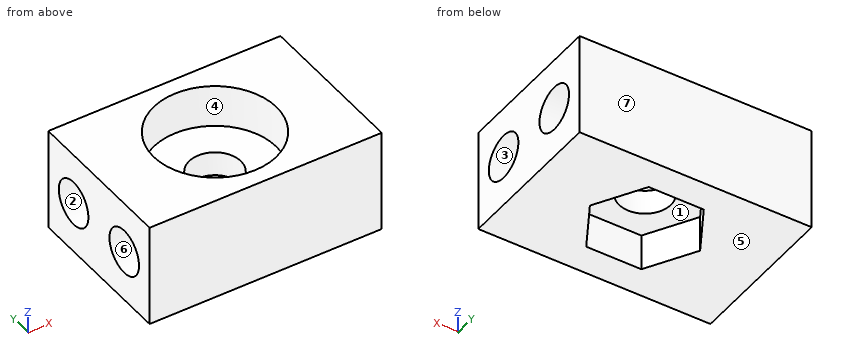
Autodesk Fusion 360 part; units mm, degrees
sketch "Sketch1" plane through (0, 0, 0) normal (0, 0, 1) x (1, 0, 0)
  line L0 (-9, -6) -> (9, -6)
  line L1 (9, -6) -> (9, 6)
  line L2 (9, 6) -> (-9, 6)
  line L3 (-9, 6) -> (-9, -6)
  dimension "d1" = 18
  dimension "d2" = 12
  dimension "d5" = 9
  dimension "d6" = 6
extrude "Extrude1" add sketch "Sketch1" along normal blind 8
sketch "Sketch2" plane through (0, 0, 0) normal (0, 0, -1) x (1, 0, 0)
  line L0 (-9, 6) -> (-9, -6)
  line L1 (-9, -6) -> (9, -6)
  line L2 (9, -6) -> (9, 6)
  line L3 (9, 6) -> (-9, 6)
sketch "Sketch3" plane through (0, 0, 0) normal (0, 0, -1) x (1, 0, 0)
  line L0 (2.1362, -3.7) -> (4.2724, 0)
  line L1 (4.2724, 0) -> (2.1362, 3.7)
  line L2 (2.1362, 3.7) -> (-2.1362, 3.7)
  line L3 (-2.1362, 3.7) -> (-4.2724, 0)
  line L4 (-4.2724, 0) -> (-2.1362, -3.7)
  line L5 (-2.1362, -3.7) -> (2.1362, -3.7)
  dimension "d12" = 3.7
extrude "Extrude2" cut sketch "Sketch3" against normal blind 2.8
sketch "Sketch4" plane through (0, 0, 8) normal (0, 0, 1) x (-1, 0, 0)
  line L0 (9, -6) -> (9, 6)
  line L1 (9, 6) -> (-9, 6)
  line L2 (-9, 6) -> (-9, -6)
  line L3 (-9, -6) -> (9, -6)
  circle A0 centre (0, 0) radius 2
  dimension "d9" = 4
extrude "Extrude3" cut sketch "Sketch4" against normal blind 10 contours A0
sketch "Sketch5" plane through (0, 0, 8) normal (0, 0, 1) x (-1, 0, 0)
  circle A0 centre (0, 0) radius 2
  line L0 (9, -6) -> (9, 6)
  line L1 (9, 6) -> (-9, 6)
  line L2 (-9, 6) -> (-9, -6)
  line L3 (-9, -6) -> (9, -6)
  circle A1 centre (0, 0) radius 4.75
  dimension "d21" = 9.5
extrude "Extrude4" cut sketch "Sketch5" against normal blind 3.3 contours A1
sketch "Sketch6" plane through (9, 0, 0) normal (1, 0, 0) x (0, 1, 0)
  line L0 (-6, 0) -> (6, 0)
  line L1 (6, 0) -> (6, 8)
  line L2 (6, 8) -> (-6, 8)
  line L3 (-6, 8) -> (-6, 0)
  line L4 (-6, 4) -> (6, 4) construction
  circle A0 centre (-3, 4) radius 1.75
  circle A1 centre (3, 4) radius 1.75
  dimension "d15" = 3.5
  dimension "d16" = 3.5
  dimension "d17" = 3
  dimension "d18" = 3
extrude "Extrude5" cut sketch "Sketch6" against normal blind 4.2 contours A0 | A1
sketch "Sketch7" plane through (-9, 0, 0) normal (-1, 0, 0) x (0, -1, 0)
  line L0 (-6, 0) -> (6, 0)
  line L1 (6, 0) -> (6, 8)
  line L2 (6, 8) -> (-6, 8)
  line L3 (-6, 8) -> (-6, 0)
  line L4 (-6, 4) -> (6, 4) construction
  circle A0 centre (-3, 4) radius 1.75
  circle A1 centre (3, 4) radius 1.75
  dimension "d24" = 3.5
  dimension "d25" = 3.5
  dimension "d26" = 3
  dimension "d27" = 3
extrude "Extrude6" cut sketch "Sketch7" against normal blind 4.2 contours A0 | A1
Could you check a few things on this model? Use its own coordinates, in mm. Face numbers are marked on the shaded views. A direction names the side the tool comes from. Give positions to 0.01 mm unless a question says otherwise; leave off trailing zeros. Loops run counter-clockwise (first coordinate to the right, second up) from the corner with the lowest first, then second, coordinate; pieces in that order, holes last. Notation, with made-up numbers: (39, 85.25) -> (91, 85.25) arc R12 ccw to (91, 97.25) -> close; hole circle Ø3 at (84.5, 56). An arc over 180 degrees is marked (long way). Return JSON: item names as keys, results as strings.
Item 1: If we section it at A-A on z = 4: List the corners of the cut face in (x, y) for me, plus the area to 3 significant figures.
Geometry results:
{"outline": "(-9, -6) -> (9, -6) -> (9, -4.75) -> (4.8, -4.75) -> (4.8, -1.25) -> (9, -1.25) -> (9, 1.25) -> (4.8, 1.25) -> (4.8, 4.75) -> (9, 4.75) -> (9, 6) -> (-9, 6) -> (-9, 4.75) -> (-4.8, 4.75) -> (-4.8, 1.25) -> (-9, 1.25) -> (-9, -1.25) -> (-4.8, -1.25) -> (-4.8, -4.75) -> (-9, -4.75) -> close; hole circle Ø4 at (0, 0)", "area": "145 mm²"}
Item 2: If we section it at D-D on x = -5.25: List the corners of the cut face in (y, z) for me.
Geometry results:
{"outline": "(-6, 0) -> (6, 0) -> (6, 8) -> (-6, 8) -> close; hole circle Ø3.5 at (-3, 4); hole circle Ø3.5 at (3, 4)"}
Item 3: If we section it at C-C on y = 0.25: List the corners of the cut face in (x, z) for me.
Geometry results:
{"outline": "(-9, 0) -> (-4.13, 0) -> (-4.13, 2.8) -> (-1.98, 2.8) -> (-1.98, 4.7) -> (-4.74, 4.7) -> (-4.74, 8) -> (-9, 8) -> close; (1.98, 2.8) -> (4.13, 2.8) -> (4.13, 0) -> (9, 0) -> (9, 8) -> (4.74, 8) -> (4.74, 4.7) -> (1.98, 4.7) -> close"}
Item 4: Which directions (+Z, -Z, +X, -X, +Y, -Y) give clear straight access to the entire face, cutting with the end or side of a thin tool? Please do the marked faces 1, 2, 3 and 4.
Geometry results:
{"face 1": "-Z", "face 2": "-X", "face 3": "+X", "face 4": "+Z"}
Item 5: If we section it at B-B on x = 0: List the corners of the cut face in (y, z) for me.
Geometry results:
{"outline": "(-6, 0) -> (-3.7, 0) -> (-3.7, 2.8) -> (-2, 2.8) -> (-2, 4.7) -> (-4.75, 4.7) -> (-4.75, 8) -> (-6, 8) -> close; (2, 2.8) -> (3.7, 2.8) -> (3.7, 0) -> (6, 0) -> (6, 8) -> (4.75, 8) -> (4.75, 4.7) -> (2, 4.7) -> close"}
Item 6: I need wall thicknesses on L1, parallel to Z at x = 7.15, y = 3; L2, parallel to Y at x = 0, z = 7.15; L3, parallel to Y at x = 0, z = 4. Which ranges of each line are inside material? Lowest first, please. Write a range as from..to.
Geometry results:
{"L1": "z = 0..2.25, 5.75..8", "L2": "y = -6..-4.75, 4.75..6", "L3": "y = -6..-2, 2..6"}
Item 7: We'd pull the mould along Y, two halves only. Please class the marked faces 5, 6 and 7: +Y half, -Y half, draft (parallel to the pull), parting line (faces both ways), or undercut.
Geometry results:
{"face 5": "draft", "face 6": "undercut", "face 7": "+Y half"}
Item 8: I'm going to push flat-ended pins straight in: pin 1 (3 mm diameter, centred on y = 3, z = 4, fed in from -X); pin 2 (2.5 mm diameter, centred on x = 0, y = 0, fed in from +Z); pin 3 (3 mm diameter, centred on y = 3, z = 4, fed in from +X). Where does each tip first touch, or does it pass through?
Geometry results:
{"pin 1": "stops at x = -4.8", "pin 2": "passes through", "pin 3": "stops at x = 4.8"}
